from build123d import *

# Parameters (mm, degrees)
F0_W     = 140
F0_H     = 23.5
F1_DEPTH = 50
F2_R     = 11.74999
F3_R     = 5
F4_DEPTH = 140
F6_DEPTH = 25
F7_W     = 140
F7_H     = 23.5
F8_DEPTH = 50


# Not quite as in the source:
# - a fillet or chamfer is up to 0.001 mm smaller than in the source, because OpenCascade refuses the exact size


with BuildPart() as f1:
    # F0 (on Front) → F1 (new body)
    with BuildSketch(Plane.XZ):
        with Locations((-8.7296748534, -19.8372076215)):
            Rectangle(F0_W, F0_H)
    extrude(amount=F1_DEPTH)

    # F2 (radius 11.75 in the source; OpenCascade refuses exactly that, so slightly less here)
    f2_edges = [f1.edges().sort_by_distance(p)[0] for p in [
        (-8.729675, -50, -8.087208),
        (-8.729675, -50, -31.587208),
    ]]
    fillet(f2_edges, radius=F2_R)

    # F3 (on face) → F4 (cut, through all)
    with BuildSketch(Plane(origin=(-78.7296748534, 0, 0), x_dir=(0, -1, 0), z_dir=(-1, 0, 0))):
        with Locations((38.25, -19.8372076215)):
            Circle(F3_R)
    extrude(amount=-F4_DEPTH, mode=Mode.SUBTRACT)

    # F5 (on face) → F6 (cut)
    with BuildSketch(Plane(origin=(0, 0, -31.5872076215), x_dir=(1, 0, 0), z_dir=(0, 0, -1))):
        Polygon((-48.7296748534, 26.5), (-48.7296748534, 51.5), (-48.7296748534, 66.3150921464), (-82.7311202884, 66.3150921464), (-82.7311202884, 26.5), (-78.7296748534, 26.5), align=None)
        Polygon((31.2703251466, 61.9400218129), (31.2703251466, 51.5), (31.2703251466, 26.5), (74.6265202761, 26.5), (74.6265202761, 61.9400218129), align=None)
    extrude(amount=-F6_DEPTH, mode=Mode.SUBTRACT)

    # F7 (on face) → F8 (join)
    with BuildSketch(Plane(origin=(0, 0, 0), x_dir=(-1, 0, 0), z_dir=(0, 1, 0))):
        with Locations((8.7296748534, -19.8372076215)):
            Rectangle(F7_W, F7_H)
    extrude(amount=F8_DEPTH)


solid = f1.part
Read the model definition and answer for the solid it produces. Units are mm, in the model's axes. A direction names the side the tool comes from. Coordinates: 2 decimals unless noted, no trailing zeros. Loops run counter-clockwise (first coordinate to the right, second up) from the corner with the lowest first, then second, coordinate; pieces in that order, holes last. Notation, with made-up numbers: (52.25, 30.25) -> (72.25, 30.25) arc R29 cw to (72.25, 54.25) -> close; hole circle Ø8 at (29.25, 89). An arc over 180 degrees is marked (long way). Write item = value, one per line. Start each with the question number.
1) The part is cut by section C-C, the plane x = 34.5. Determine the outline of the cut face in (y, z), plus the area to 3 significant figures.
2) The mould has two halves that part along Y. Classify faces 1 (the face through (-8.17, -46.467, -28.237)), 2 (the face through (-9.29, -34.565, -16.458)), 3 (the face through (31.27, -33, -20)): pulls with the +Y half, pulls with the -Y half, needs draft (parallel to the pull), parting line crosses it, or undercut.
3) Given P1, Ø13, axis at y = -38.25, z = -19.84, coming from the +X side; P2, Ø12, axis at y = -36, z = -23, coming from the -X side; P3, Ø12, axis at x = -68.5, z = -17.5, coming from the -Y side, each flat-ended and moving along its own axis, determine where each tip first touches the part or whether it passes through.
4) The part is cut by section A-A, the plane z = -22.5. Determine the outline of the cut face in (x, y), plus the area to 3 significant figures.
5) Find the intervals of material crossed by L1, parallel to Z at x = -27.5, y = -38.25; L2, parallel to Y at x = 33, z = -24.5; L3, parallel to X at y = -28, z = -19.25, in increasing order. Write a range as from..to.
6) The part is cut by section B-B, the plane y = -41. Determine the outline of the cut face in (x, z), plus the area to 3 significant figures.
7) The part is cut by section D-D, the plane z = -12.25. Determine the outline of the cut face in (x, y), plus the area to 3 significant figures.
8) For faces 4 (the face through (-48.73, -33, -20)), 5 (the face through (-8, 5, -31.587)), 6 (the face through (46, -26.5, -20)), determine the directions among +Z, -Z, +X, -X, +Y, -Y from which every point of the face is accessible in a straight line to the end or side of a thin tool.
Result:
q1.outline = (-26.5, -31.59) -> (50, -31.59) -> (50, -8.09) -> (-26.5, -8.09) -> close
q1.area = 1,800 mm²
q2.face_1 = pulls with the -Y half
q2.face_2 = undercut
q2.face_3 = needs draft
q3.P1 = 31.27
q3.P2 = -48.73
q3.P3 = -26.5
q4.outline = (-78.73, -26.5) -> (-48.73, -26.5) -> (-48.73, -34.02) -> (31.27, -34.02) -> (31.27, -26.5) -> (61.27, -26.5) -> (61.27, 50) -> (-78.73, 50) -> close; (-48.73, -49.69) -> (31.27, -49.69) -> (31.27, -42.48) -> (-48.73, -42.48) -> close
q4.area = 11,900 mm²
q5.L1 = -31.59..-24.84, -14.84..-8.09
q5.L2 = -26.5..50
q5.L3 = -48.73..31.27
q6.outline = (-48.73, -31.26) -> (31.27, -31.26) -> (31.27, -24.01) -> (-48.73, -24.01) -> close; (-48.73, -15.66) -> (31.27, -15.66) -> (31.27, -8.41) -> (-48.73, -8.41) -> close
q6.area = 1,160 mm²
q7.outline = (-78.73, -26.5) -> (-48.73, -26.5) -> (-48.73, -47.22) -> (31.27, -47.22) -> (31.27, -26.5) -> (61.27, -26.5) -> (61.27, 50) -> (-78.73, 50) -> close
q7.area = 12,400 mm²
q8.face_4 = +Z, -Z, -X, -Y
q8.face_5 = -Z, +X, -X, +Y, -Y
q8.face_6 = +Z, -Z, +X, -Y
